```python
from build123d import *

# Parameters (mm, degrees)
SKETCH1_W           = 88
SKETCH1_H           = 88
BOSS_EXTRUDE1_DEPTH = 5
FILLET1_R           = 10
SKETCH2_R           = 2.15
CUT_EXTRUDE1_DEPTH  = 63.42595614
SKETCH3_W           = 4
SKETCH3_H           = 50
BOSS_EXTRUDE2_DEPTH = 10
CHAMFER1_SIZE       = 10
SKETCH4_R           = 1.5
CUT_EXTRUDE2_DEPTH  = 65.007812023
SKETCH5_R           = 3.5
CUT_EXTRUDE3_DEPTH  = 7.5
CUT_EXTRUDE4_START  = -7.5
SKETCH6_R           = 3.5
CUT_EXTRUDE4_DEPTH  = 7.5
LPATTERN2_COUNT     = 5
LPATTERN2_PITCH     = 10
CHAMFER2_SIZE       = 6
SKETCH7_R           = 25
CUT_EXTRUDE5_DEPTH  = 64.023805026
SKETCH8_R           = 4
CUT_EXTRUDE6_DEPTH  = 64.023805026


with BuildPart() as part:
    # Sketch1 → Boss-Extrude1 (new body)
    with BuildSketch(Plane(origin=(0, 0, 0), x_dir=(1, 0, 0), z_dir=(0, 1, 0))):
        Rectangle(SKETCH1_W, SKETCH1_H)
    extrude(amount=BOSS_EXTRUDE1_DEPTH)

    # Fillet1
    fillet1_edges = [part.edges().sort_by_distance(p)[0] for p in [
        (-44, 2.5, -44),
        (44, 2.5, -44),
        (44, 2.5, 44),
        (-44, 2.5, 44),
    ]]
    fillet(fillet1_edges, radius=FILLET1_R)

    # Sketch2 → Cut-Extrude1 (cut, through all)
    with BuildSketch(Plane(origin=(0, 5, 0), x_dir=(1, 0, 0), z_dir=(0, 1, 0))):
        with Locations(Location((34, 34, 0), (0, 0, 270))):
            Circle(SKETCH2_R)
        with Locations(Location((34, -34, 0), (0, 0, 270))):
            Circle(SKETCH2_R)
        with Locations(Location((-34, -34, 0), (0, 0, 270))):
            Circle(SKETCH2_R)
        with Locations(Location((-34, 34, 0), (0, 0, 270))):
            Circle(SKETCH2_R)
    extrude(amount=-CUT_EXTRUDE1_DEPTH, mode=Mode.SUBTRACT)

    # Sketch3 → Boss-Extrude2 (add)
    with BuildSketch(Plane(origin=(0, 5, 0), x_dir=(1, 0, 0), z_dir=(0, 1, 0))):
        with Locations((-35.5, 0)):
            Rectangle(SKETCH3_W, SKETCH3_H)
        with Locations((35.5, 0)):
            Rectangle(SKETCH3_W, SKETCH3_H)
    extrude(amount=BOSS_EXTRUDE2_DEPTH)

    # Chamfer1
    # the kernel refuses this chamfer: 10 mm, written as the material it adds along each edge
    with BuildSketch(Plane(origin=(37.5, 5, 25), x_dir=(0.9996219169112968, -0.027495876610586403, 0), z_dir=(0, 0, -1))) as chamfer1_piece_1_section:
        Polygon((CHAMFER1_SIZE * 0.999621916911, -CHAMFER1_SIZE * 0.0274958766106), (-CHAMFER1_SIZE * 0.0274958766106, -CHAMFER1_SIZE * 0.999621916911), (0, 0), align=None)
    chamfer1_piece_1 = extrude(amount=50, mode=Mode.PRIVATE)
    chamfer1_piece_1 = split(chamfer1_piece_1, bisect_by=Plane(origin=(44, 8.634022107, 0), z_dir=(-1, 0, 0)), keep=Keep.TOP, mode=Mode.PRIVATE)
    add(chamfer1_piece_1)
    with BuildSketch(Plane(origin=(-37.5, 5, -25), x_dir=(-0.9996219169112968, -0.027495876610586403, 0), z_dir=(0, 0, 1))) as chamfer1_piece_2_section:
        Polygon((CHAMFER1_SIZE * 0.999621916911, -CHAMFER1_SIZE * 0.0274958766106), (-CHAMFER1_SIZE * 0.0274958766106, -CHAMFER1_SIZE * 0.999621916911), (0, 0), align=None)
    chamfer1_piece_2 = extrude(amount=50, mode=Mode.PRIVATE)
    chamfer1_piece_2 = split(chamfer1_piece_2, bisect_by=Plane(origin=(-44, 8.634022107, 0), z_dir=(1, 0, 0)), keep=Keep.TOP, mode=Mode.PRIVATE)
    add(chamfer1_piece_2)

    # Sketch4 → Cut-Extrude2 (cut, symmetric)
    with BuildSketch(Plane(origin=(0, 0, 0), x_dir=(0, 0, -1), z_dir=(1, 0, 0))):
        with Locations(Location((-20, 9, 0), (0, 0, 340.528779366))):
            Circle(SKETCH4_R)
    cut_extrude2 = extrude(amount=CUT_EXTRUDE2_DEPTH, both=True, mode=Mode.SUBTRACT)

    # Sketch5 → Cut-Extrude3 (cut)
    with BuildSketch(Plane(origin=(44, 0, 0), x_dir=(0, 0, -1), z_dir=(1, 0, 0))):
        with Locations((-20, 9)):
            Circle(SKETCH5_R)
    cut_extrude3 = extrude(amount=-CUT_EXTRUDE3_DEPTH, mode=Mode.SUBTRACT)

    # Sketch6 → Cut-Extrude4 (cut)
    with BuildSketch(Plane.ZY.offset(44).offset(CUT_EXTRUDE4_START)):
        with Locations(Location((20, 9, 0), (0, 0, 180))):
            Circle(SKETCH6_R)
    cut_extrude4 = extrude(amount=CUT_EXTRUDE4_DEPTH, mode=Mode.SUBTRACT)

    # LPattern2: Cut-Extrude2, Cut-Extrude3, Cut-Extrude4 ×5
    with Locations(*[(0, 0, -i * LPATTERN2_PITCH) for i in range(1, LPATTERN2_COUNT)]):
        add(cut_extrude2, mode=Mode.SUBTRACT)
        add(cut_extrude3, mode=Mode.SUBTRACT)
        add(cut_extrude4, mode=Mode.SUBTRACT)

    # Chamfer2
    # the kernel refuses this chamfer: 6 mm, written as the material it adds along each edge
    with BuildSketch(Plane(origin=(-44, 5, 25), x_dir=(-2.4740283856501726e-13, 0.9996219169112965, -0.027495876610592693), z_dir=(1, 0, 0))) as chamfer2_piece_1_section:
        Polygon((CHAMFER2_SIZE * 0.999621916911, CHAMFER2_SIZE * 0.0274958766106), (-CHAMFER2_SIZE * 0.0274958766102, CHAMFER2_SIZE * 0.999621916911), (0, 0), align=None)
    chamfer2_piece_1 = extrude(amount=10.5, mode=Mode.PRIVATE)
    chamfer2_piece_1 = split(chamfer2_piece_1, bisect_by=Plane(origin=(-42.122041118, 10.377958882, 27.00389647), z_dir=(0.7071067811868302, -0.7071067811862648, 0)), keep=Keep.TOP, mode=Mode.PRIVATE)
    add(chamfer2_piece_1)
    with BuildSketch(Plane(origin=(-33.5, 5, -25), x_dir=(-2.474214452272925e-13, 0.9996219169112968, 0.027495876610585616), z_dir=(-1, 0, 0))) as chamfer2_piece_2_section:
        Polygon((CHAMFER2_SIZE * 0.999621916911, CHAMFER2_SIZE * 0.0274958766106), (-CHAMFER2_SIZE * 0.0274958766106, CHAMFER2_SIZE * 0.999621916911), (0, 0), align=None)
    chamfer2_piece_2 = extrude(amount=10.5, mode=Mode.PRIVATE)
    chamfer2_piece_2 = split(chamfer2_piece_2, bisect_by=Plane(origin=(-42.122041118, 10.377958882, -27.00389647), z_dir=(0.7071067811868302, -0.7071067811862648, 0)), keep=Keep.TOP, mode=Mode.PRIVATE)
    add(chamfer2_piece_2)
    with BuildSketch(Plane(origin=(44, 5, -25), x_dir=(5.708966314845366e-15, -0.027495876610159536, -0.9996219169113084), z_dir=(-1, 0, 0))) as chamfer2_piece_3_section:
        Polygon((CHAMFER2_SIZE * 0.999621916911, -CHAMFER2_SIZE * 0.0274958766106), (-CHAMFER2_SIZE * 0.0274958766102, -CHAMFER2_SIZE * 0.999621916911), (0, 0), align=None)
    chamfer2_piece_3 = extrude(amount=10.5, mode=Mode.PRIVATE)
    chamfer2_piece_3 = split(chamfer2_piece_3, bisect_by=Plane(origin=(42.122041118, 10.377958882, -27.00389647), z_dir=(-0.7071067811868302, -0.7071067811862648, 0)), keep=Keep.TOP, mode=Mode.PRIVATE)
    add(chamfer2_piece_3)
    with BuildSketch(Plane(origin=(33.5, 5, 25), x_dir=(-1.864328825330305e-14, -0.02749587661058664, 0.9996219169112968), z_dir=(1, 0, 0))) as chamfer2_piece_4_section:
        Polygon((CHAMFER2_SIZE * 0.999621916911, -CHAMFER2_SIZE * 0.0274958766106), (-CHAMFER2_SIZE * 0.0274958766106, -CHAMFER2_SIZE * 0.999621916911), (0, 0), align=None)
    chamfer2_piece_4 = extrude(amount=10.5, mode=Mode.PRIVATE)
    chamfer2_piece_4 = split(chamfer2_piece_4, bisect_by=Plane(origin=(42.122041118, 10.377958882, 27.00389647), z_dir=(-0.7071067811868302, -0.7071067811862648, 0)), keep=Keep.TOP, mode=Mode.PRIVATE)
    add(chamfer2_piece_4)

    # Sketch7 → Cut-Extrude5 (cut, through all)
    with BuildSketch(Plane(origin=(0, 5, 0), x_dir=(1, 0, 0), z_dir=(0, 1, 0))):
        with Locations(Location((0, 0, 0), (0, 0, 270))):
            Circle(SKETCH7_R)
    extrude(amount=-CUT_EXTRUDE5_DEPTH, mode=Mode.SUBTRACT)

    # Sketch8 → Cut-Extrude6 (cut, through all)
    with BuildSketch(Plane(origin=(0, 5, 0), x_dir=(1, 0, 0), z_dir=(0, 1, 0))):
        with Locations((-34, -34)):
            Circle(SKETCH8_R)
        with Locations((34, -34)):
            Circle(SKETCH8_R)
        with Locations((34, 34)):
            Circle(SKETCH8_R)
        with Locations((-34, 34)):
            Circle(SKETCH8_R)
    extrude(amount=CUT_EXTRUDE6_DEPTH, mode=Mode.SUBTRACT)


solid = part.part
```
Design review of the part built by this model. Coordinates are the model's own, in mm. A direction names the side the tool comes from. Coordinates: 2 decimals unless noted, no trailing zeros. Loops run counter-clockwise (first coordinate to the right, second up) from the corner with the lowest first, then second, coordinate; pieces in that order, holes last.
Q1. We need section D-D on x = 0. State the section outline as (y, z) points.
Reported:
outline: (0, -44) - (5, -44) - (5, -25) - (0, -25) - close; (0, 25) - (5, 25) - (5, 44) - (0, 44) - close
Q2. The part is to be moulded in two halves that separate along X. For faces 1 (the face through (-32.19, 2.54, -32.84)), 2 (the face through (-34.979, 10.467, -20.312)), 3 (the face through (-44, 3, 0)), say which applies: +X half, -X half, draft (parallel to the pull), parting line (faces both ways), or undercut.
Reported:
face 1: undercut
face 2: draft
face 3: -X half
Q3. Tool access review of faces 4 (the face through (-36, 15, 0)), 5 (the face through (39.469, 5.583, 10.759)), 6 (the face through (37, 13, -25)), 7 (the face through (-39.36, 5.53, -19.54)): name each direction out of +Z, -Z, +X, -X, +Y, -Y from which nothing blocks a thin tool from reaching the whole face with its end or side.
Reported:
face 4: +Z, -Z, +X, -X, +Y
face 5: +X
face 6: -Z, +X, -X, +Y
face 7: -X
Q4. We need section A-A on z = 20. State the section outline as (x, y) points, and give its area (3 significant figures).
Reported:
outline: (-44, 0) - (-15, 0) - (-15, 5) - (-33.5, 5) - (-33.5, 7.5) - (-36.5, 7.5) - (-36.5, 5.5) - (-44, 5.5) - close; (-40, 12.5) - (-36.5, 12.5) - (-36.5, 10.5) - (-33.5, 10.5) - (-33.5, 15) - (-37.5, 15) - close; (15, 0) - (44, 0) - (44, 5.5) - (36.5, 5.5) - (36.5, 7.5) - (33.5, 7.5) - (33.5, 5) - (15, 5) - close; (33.5, 10.5) - (36.5, 10.5) - (36.5, 12.5) - (40, 12.5) - (37.5, 15) - (33.5, 15) - close
area: 351 mm2
Q5. We need section B-B on x = -15. State the section outline as (y, z) points, and give its area (3 significant figures).
Reported:
outline: (0, -44) - (5, -44) - (5, -20) - (0, -20) - close; (0, 20) - (5, 20) - (5, 44) - (0, 44) - close
area: 240 mm2
Q6. To check wall thickness, follow line 1 (X direction, y = 11, z = -11); line 2 (X direction, y = 1.5, z = 34); line 3 (Y direction, x = -34.75, z = 20). State the ranges of each line that lie inside material, in increasing order.
Reported:
line 1: x = -36.5 to -33.5, 33.5 to 36.5
line 2: x = -44 to -36.15, -31.85 to 31.85, 36.15 to 44
line 3: y = 0 to 7.5, 10.5 to 15
Q7. For pin 1 (2 mm diameter, centred on x = 37, y = 13, fed in from -Z); pin 2 (2 mm diameter, centred on x = 12, z = -33.5, fed in from +Y); pin 3 (3.5 mm diameter, centred on y = 9, z = -20, fed in from -X); pin 4 (2.5 mm diameter, centred on x = -34, z = -34, fed in from +Y), all flat-tipped, find the tip position at first contact; note any pin that passes through.
Reported:
pin 1: stops at z = -25
pin 2: stops at y = 5
pin 3: stops at x = -36.5
pin 4: passes through
Q8. We need section C-C on y = 3.25. State the section outline as (x, z) points.
Reported:
outline: (-44, -34) arc R10 ccw to (-34, -44) - (34, -44) arc R10 ccw to (44, -34) - (44, 34) arc R10 ccw to (34, 44) - (-34, 44) arc R10 ccw to (-44, 34) - close; hole circle Ø4.3 at (-34, -34); hole circle Ø4.3 at (-34, 34); hole circle Ø50 at (0, 0); hole circle Ø4.3 at (34, -34); hole circle Ø4.3 at (34, 34)
